from build123d import *

# Parameters (mm, degrees)
F1_DEPTH = 25
F2_DEPTH = 40
F3_D     = 15
F4_D     = 15


with BuildPart() as f1:
    # F0 (on Front) → F1 (new body)
    with BuildSketch(Plane.XZ):
        Polygon((-77.238509, -21.429978), (-52.238509, -64.731248), (-27.238509, -21.429978), (-52.238509, -21.429978), align=None)
    extrude(amount=-F1_DEPTH)

    # F0 (on Front) → F2 (join)
    with BuildSketch(Plane.XZ):
        Polygon((-102.238509, -21.429978), (-77.238509, -21.429978), (-52.238509, -21.429978), (-27.238509, -21.429978), (-39.738509, 0.220657), (-52.238509, 0.220657), (-89.738509, 0.220657), align=None)
    extrude(amount=-F2_DEPTH)

    # F3 (through all)
    with Locations(Plane.XZ):
        with Locations((-52.238509, -10.60466)):
            Hole(F3_D / 2)

    # F4 (through all)
    with Locations(Plane.XZ):
        with Locations((-77.238509, -10.60466)):
            Hole(F4_D / 2)


solid = f1.part
Check sheet for the modelled part. Datum: model origin and axes. Units: mm. A direction names the side the tool comes from. Give positions to 0.01 mm unless a question says otherwise; leave off trailing zeros. Loops run counter-clockwise (first coordinate to the right, second up) from the corner with the lowest first, then second, coordinate; pieces in that order, holes last. Notation, with made-up numbers: M 87,65 L 140,65 A18 ccw 140,86 Z; hole C 72,-37 d9. An arc over 180 degrees is marked long. Return JSON: item names as keys, results as strings. Group by question number.
1. Cross-section at B-B on y = 16.5. Record the boundary of the cut face in (x, z).
2. Cross-section at A-A on z = -11.5. Record the boundary of the cut face in (x, y).
3. Mould release check, pull along X, two halves, no side actions. Record for faces 4 (the flat face through (-95.9, 19.72, -10.45)), 5 (the flat face through (-65, 40, -10)), 6 (the cylindrical face through (-69.746, 20.28, -10.275)): released by +X, released by -X, zero draft, split by the parting line, or undercut.
4. Thickness scan on L1, parallel to X at y = 6, z = -5.5; L2, parallel to X at y = 26, z = -8; L3, parallel to Y at x = -67.5, z = -25. Record the ranges inside material, lowest first.
5. Go/stop test with flat-tipped pins: pin 1 (3 mm diameter, centred on y = 9.5, z = -32, fed in from +X); pin 2 (21.5 mm diameter, centred on x = -41, z = -36.5, fed in from +Y); pin 3 (1 mm diameter, centred on y = 17, z = -39.5, fed in from +X); pin 4 (8 mm diameter, centred on x = -77.5, z = -9.5, fed in from +Y). Record where each tip stops, or that it passes through.
6. Cross-section at D-D on x = -65. Record the boundary of the cut face in (y, z), plus the area to 3 significant figures.
7. Tool access check on faces 1 (the flat face through (-74, 29, -21.43)), 2 (the flat face through (-64, 20, 0.221)), 3 (the flat face through (-53, 25, -38)). Record the directions out of +Z, -Z, +X, -X, +Y, -Y that give a thin tool (end or side, any length) a straight path to the whole face; none if there is none.
8. Cross-section at C-C on x = -81. Record the boundary of the cut face in (y, z).
Return value:
{
 "1": {"outline": "M -102.24,-21.43 L -77.24,-21.43 L -52.24,-64.73 L -27.24,-21.43 L -39.74,0.22 L -89.74,0.22 Z; hole C -77.24,-10.6 d15; hole C -52.24,-10.6 d15"},
 "2": {"outline": "M -96.51,0 L -84.68,0 L -84.68,40 L -96.51,40 Z; M -69.79,0 L -59.68,0 L -59.68,40 L -69.79,40 Z; M -44.79,0 L -32.97,0 L -32.97,40 L -44.79,40 Z"},
 "3": {"face 4": "released by -X", "face 5": "zero draft", "face 6": "undercut"},
 "4": {"L1": "-93.04 to -82.73, -71.74 to -57.73, -46.74 to -36.44", "L2": "-94.48 to -84.27, -70.21 to -59.27, -45.21 to -34.99", "L3": "0 to 25"},
 "5": {"pin 1": "x = -32.48", "pin 2": "y = 25", "pin 3": "x = -37.38", "pin 4": "through"},
 "6": {"outline": "M 0,-42.63 L 25,-42.63 L 25,-21.43 L 40,-21.43 L 40,0.22 L 0,0.22 Z", "area": "1,400 mm^2"},
 "7": {"face 1": "-Z, -X, +Y", "face 2": "+Z, +X, -X, +Y, -Y", "face 3": "-Z, +X, -X, +Y"},
 "8": {"outline": "M 0,-21.43 L 40,-21.43 L 40,-17.09 L 0,-17.09 Z; M 0,-4.12 L 40,-4.12 L 40,0.22 L 0,0.22 Z"}
}
